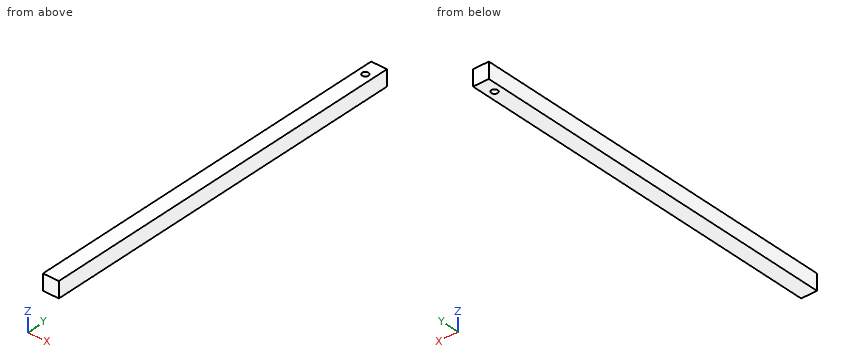
```python
from build123d import *

# Parameters (mm, degrees)
SKETCH1_W           = 5
SKETCH1_H           = 120
BOSS_EXTRUDE1_DEPTH = 5
SKETCH2_R           = 1
CUT_EXTRUDE1_DEPTH  = 10


with BuildPart() as part:
    # Sketch1 → Boss-Extrude1 (new body)
    with BuildSketch(Plane.XY):
        with Locations((0, 60)):
            Rectangle(SKETCH1_W, SKETCH1_H)
    extrude(amount=BOSS_EXTRUDE1_DEPTH)

    # Sketch2 → Cut-Extrude1 (cut, symmetric)
    with BuildSketch(Plane.XY):
        with Locations((0, 115)):
            Circle(SKETCH2_R)
    extrude(amount=CUT_EXTRUDE1_DEPTH, both=True, mode=Mode.SUBTRACT)


solid = part.part
```
Geometry: final body of the model. Coordinates: model frame, mm. Give positions to 0.01 mm unless a question says otherwise; leave off trailing zeros. Write each loop counter-clockwise with the first axis right and the second up, starting at its lowest first coordinate (ties: lowest second). Pieces come first, ordered by that corner, then holes.
1. Line query: probe 1 along X at (y, z) = (115, 2.7); probe 2 along Y at (x, z) = (0, 1.75); probe 3 along Y at (x, z) = (0.8, 3.5). Output: solid intervals per line, ascending.
2. Section query A-A, the plane x = 0. Return loops of the section in (y, z).
3. Section query B-B, the plane y = 115. Return loops of the section in (x, z), then the cut area to 3 significant figures.
Computed:
1. probe 1: x = -2.5 to -1, 1 to 2.5
1. probe 2: y = 0 to 114, 116 to 120
1. probe 3: y = 0 to 114.4, 115.6 to 120
2. outline: (0, 0) - (114, 0) - (114, 5) - (0, 5) - close; (116, 0) - (120, 0) - (120, 5) - (116, 5) - close
3. outline: (-2.5, 0) - (-1, 0) - (-1, 5) - (-2.5, 5) - close; (1, 0) - (2.5, 0) - (2.5, 5) - (1, 5) - close
3. area: 15.0 mm2
